Can you work these out from the drawing? Everything is in mm from the part's minimum corner. Give positions to 0.01 mm unless a question says otherwise; leave off trailing zeros. Order: outer loops, then holes, each group sorted by start corner. A loop starts at its lowest first (then second) coordinate and runs counter-clockwise, first axis right, second up. Notation, with made-up numbers: (-14, 9) - (22, 9) arc R7 ccw to (22, 18) - close; hole circle Ø4 at (-5.75, -31). An arc over 180 degrees is marked (long way). Answer as a JSON object with one key per item and string values.
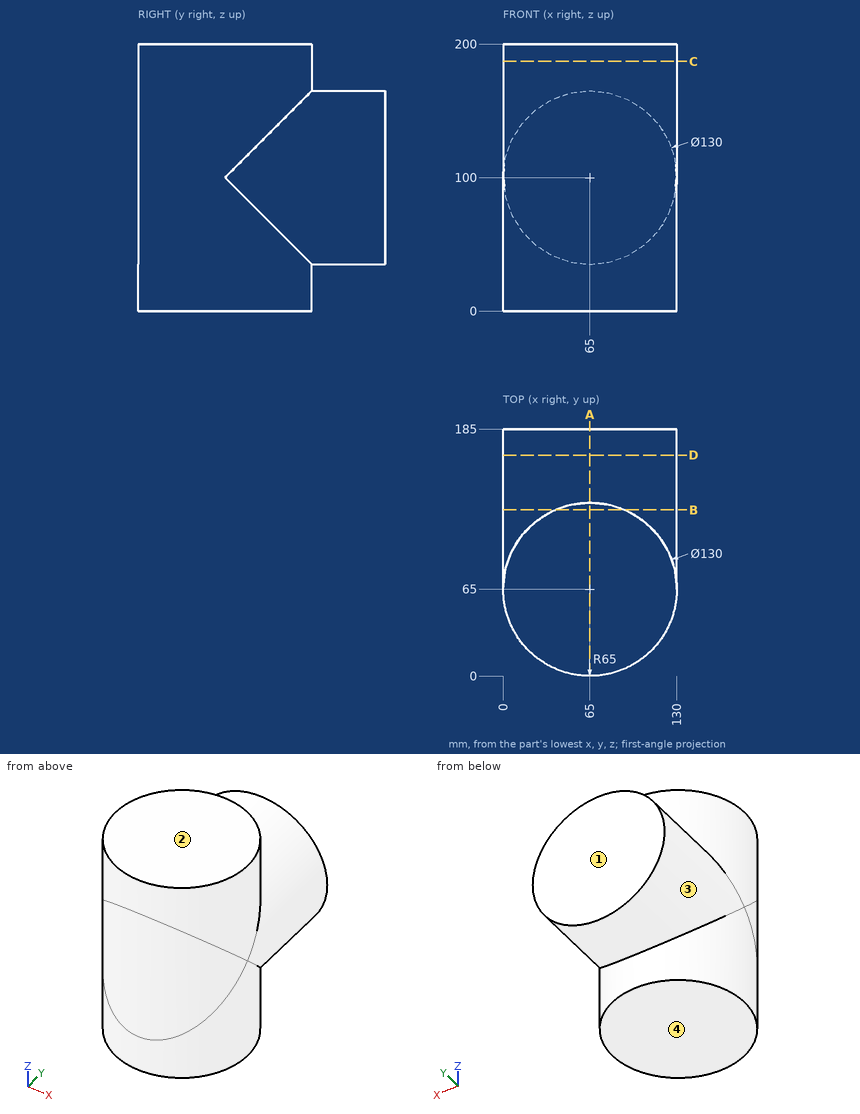
Q1. If we section it at D-D, the plane y = 165.5: Please give me the cut outline in (x, z).
Recorded:
{"outline": "circle Ø130 at (65, 100)"}
Q2. We'd pull the mould along Z, two halves only. Please class the marked faces 1, 2, 3 and 4: released by +Z, released by -Z, zero draft, split by the parting line, or undercut.
Recorded:
{"face 1": "zero draft", "face 2": "released by +Z", "face 3": "split by the parting line", "face 4": "released by -Z"}
Q3. If we section it at C-C, the plane z = 187: Please give me the cut outline in (x, y), then the cut area to 3 significant figures.
Recorded:
{"outline": "circle Ø130 at (65, 65)", "area": "13,300 mm^2"}
Q4. I'm going to push flat-ended pins straight in: pin 1 Ø3 at (y, z) = (149, 94) entering from -X; pin 2 Ø8 at (x, z) = (101, 166.5) entering from -Y; pin 3 Ø12 at (y, z) = (165, 107) entering from +X. Where does each tip first touch, or does it pass through?
Recorded:
{"pin 1": "stops at x = 0.16", "pin 2": "stops at y = 8.42", "pin 3": "stops at x = 129.99"}
Q5. I need wall thicknesses on L1, parallel to Y at x = 65, z = 180; L2, parallel to Z at x = 48, y = 128; L3, parallel to X at y = 12, z = 177. Which ranges of each line are inside material? Lowest first, please.
Recorded:
{"L1": "y = 0 to 130", "L2": "z = 37.26 to 162.74", "L3": "x = 27.37 to 102.63"}
Q6. If we section it at A-A, the plane x = 65: Please give me the cut outline in (y, z).
Recorded:
{"outline": "(0, 0) - (130, 0) - (130, 35) - (185, 35) - (185, 165) - (130, 165) - (130, 200) - (0, 200) - close"}
Q7. If we section it at B-B, the plane y = 124.5: Please give me the cut outline in (x, z), then the cut area to 3 significant figures.
Recorded:
{"outline": "(38.83, 0) - (91.17, 0) - (91.17, 40.5) arc R65 ccw to (91.17, 159.5) - (91.17, 200) - (38.83, 200) - (38.83, 159.5) arc R65 ccw to (38.83, 40.5) - close", "area": "17,100 mm^2"}
